Here's how the part is built. I have some questions about the finished solid (model axes, mm). Face numbers are marked on the shaded views. A direction names the side the tool comes from. Coordinates: 2 decimals unless noted, no trailing zeros. Write each loop counter-clockwise with the first axis right and the second up, starting at its lowest first coordinate (ties: lowest second). Pieces come first, ordered by that corner, then holes. Notation, with made-up numbers: (-11.5, -31.75) - (10.5, -31.75) arc R23 ccw to (10.5, -3.75) - close; hole circle Ø8 at (-31, 85.25). An arc over 180 degrees is marked (long way). Answer in a Markdown table with one row per item. Add a question column.
Item 1: We'd pull the mould along Z, two halves only. Please class the marked faces 3, 4 and 5: +Z half, -Z half, draft (parallel to the pull), parting line (faces both ways), or undercut.
Item 2: Imagine slicing it at B-B (z = 69). Please give me the cut outline in (x, y), plus the area to 3 significant figures.
Item 3: I'm going to push flat-ended pins straight in: pin 1 (3 mm diameter, centred on y = 13.5, z = 84, fed in from -X); pin 2 (6 mm diameter, centred on x = -2, z = 39.5, fed in from +Y) (3 decimals); pin 3 (3 mm diameter, centred on x = -6, y = -14.5, fed in from +Z). Where does each tip first touch, or does it pass through?
Item 4: Which directions (+Z, -Z, +X, -X, +Y, -Y) give clear straight access to the entire face, cutting with the end or side of a thin tool? Please do the marked faces 1 and 2.
Item 5: Imagine slicing it at A-A (z = 34). Please give me the cut outline in (x, y) (3 decimals).
Item 6: If I drill on probe 1 along X at (y, z) = (0, 72); probe 2 along X at (y, z) = (0, 31) (3 decimals), over which ranges is the centre line in solid material (lowest first)? Write a range as from..to.
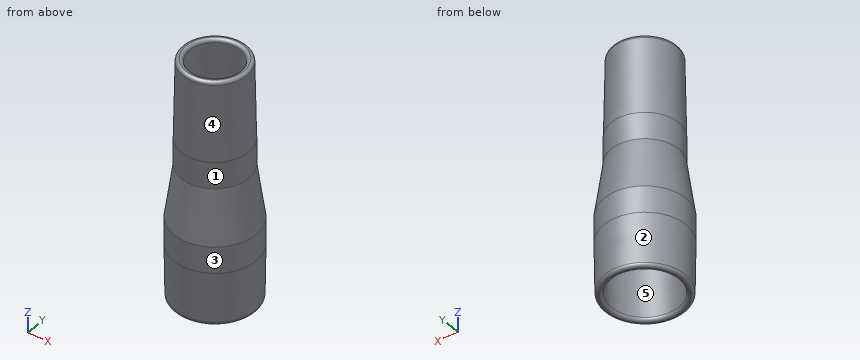
from build123d import *

# Parameters (mm, degrees)
F2_R = 1.524


with BuildPart() as f1:
    # F0 (on Front) → F1 (revolve)
    with BuildSketch(Plane.XZ):
        Polygon((-19.685, 25.4), (-19.304, 0), (-16.128643, 0), (-16.51, 25.423811), (-16.51, 37.878828), (-12.954, 63.278828), (-12.954, 76.168253), (-12.191365, 114.3), (-15.367, 114.3), (-16.129, 76.2), (-16.129, 63.5), (-19.685, 38.1), align=None)
    revolve(axis=Axis((0, 0, 60.50895), (0, 0, 1)))

    # F2
    f2_edges = [f1.edges().sort_by_distance(p)[0] for p in [
        (15.367, 0, 114.3),
        (12.191365, 0, 114.3),
        (19.304, 0, 0),
        (16.128643, 0, 0),
    ]]
    fillet(f2_edges, radius=F2_R)


solid = f1.part
Here are the results:
| question | item | result |
|---|---|---|
| 1 | face 3 | draft |
| 1 | face 4 | +Z half |
| 1 | face 5 | undercut |
| 2 | outline | circle Ø32.26 at (0, 0); hole circle Ø25.91 at (0, 0) |
| 2 | area | 290 mm2 |
| 3 | pin 1 | stops at x = -10.54 |
| 3 | pin 2 | stops at y = 19.685 |
| 3 | pin 3 | stops at z = 114.27 |
| 4 | face 1 | +Z |
| 4 | face 2 | -Z |
| 5 | outline | circle Ø39.37 at (0, 0); hole circle Ø33.02 at (0, 0) |
| 6 | probe 1 | x = -16.13..-12.95, 12.95..16.13 |
| 6 | probe 2 | x = -19.685..-16.51, 16.51..19.685 |
